Read the model definition and answer for the solid it produces. Units are mm, in the model's axes. A direction names the side the tool comes from. Give positions to 0.01 mm unless a question says otherwise; leave off trailing zeros. Order: outer loops, then holes, each group sorted by start corner. A loop starts at its lowest first (then second) coordinate and runs counter-clockwise, first axis right, second up.
```python
from build123d import *

# Parameters (mm, degrees)
F1_DEPTH      = 300
F3_DEPTH      = 473
F3_DEPTH_BACK = 473
F5_DEPTH      = 473
F5_DEPTH_BACK = 473


with BuildPart() as f1:
    # F0 (on Front) → F1 (new body)
    with BuildSketch(Plane.XZ):
        Polygon((-474, 25), (-474, 0), (473, 0), (473, 25), (472, 25), (472, 1), (-473, 1), (-473, 25), align=None)
    extrude(amount=F1_DEPTH)

    # F2 (on Right) → F3 (join, two sides)
    with BuildSketch(Plane.YZ) as f3_sk:
        with BuildLine():
            Line((-300, -30), (-300, 0))
            Line((-300, 0), (-300, 1))
            ThreePointArc((-300, 1), (-300.707107, 0.707107), (-301, 0))
            Line((-301, 0), (-301, -29))
            Line((-301, -29), (-314, -29))
            Line((-314, -29), (-314, -16))
            Line((-314, -16), (-315, -16))
            Line((-315, -16), (-315, -30))
            Line((-315, -30), (-300, -30))
        make_face()
    extrude(amount=F3_DEPTH)
    extrude(f3_sk.sketch, amount=-F3_DEPTH_BACK)

    # F4 (on Right) → F5 (join, two sides)
    with BuildSketch(Plane.YZ) as f5_sk:
        Polygon((-1, 0), (0, 0), (0, 30), (-10, 30), (-10, 20), (-9, 20), (-9, 29), (-1, 29), align=None)
    extrude(amount=F5_DEPTH)
    extrude(f5_sk.sketch, amount=-F5_DEPTH_BACK)


solid = f1.part
```
1) The part is cut by section B-B on y = -127. Determine the outline of the cut face in (x, z).
Final values:
outline: (-474, 0) - (473, 0) - (473, 25) - (472, 25) - (472, 1) - (-473, 1) - (-473, 25) - (-474, 25) - close
2) The part is cut by section A-A on x = 137. Determine the outline of the cut face in (y, z), and give its area (3 significant figures).
Final values:
outline: (-315, -30) - (-300, -30) - (-300, 0) - (0, 0) - (0, 30) - (-10, 30) - (-10, 20) - (-9, 20) - (-9, 29) - (-1, 29) - (-1, 1) - (-300, 1) arc R1 ccw to (-301, 0) - (-301, -29) - (-314, -29) - (-314, -16) - (-315, -16) - close
area: 405 mm2
3) For a pull along Z with two mould halves and no side action, classify faces 3 (the face through (7, -301, -14)), 4 (the face through (-7, -1, 15)), 5 (the face through (7, -308, -30)) as released by +Z, released by -Z, zero draft, split by the parting line, or undercut.
Final values:
face 3: zero draft
face 4: undercut
face 5: released by -Z
4) Given pin 1 (1.1 mm diameter, centred on x = 4, y = -314.5, fed in from +Z); pin 2 (0.5 mm diameter, centred on x = 472.5, y = -133.5, fed in from +Z); pin 3 (1.1 mm diameter, centred on x = 472.5, z = 7.5, fed in from -Y), each flat-ended and moving along its own axis, determine where each tip first touches the part or whether it passes through.
Final values:
pin 1: stops at z = -16
pin 2: stops at z = 25
pin 3: stops at y = -300
5) A tool of negligible diameter and unlimited length cuts with its end or side. For faces 1 (the face through (-7, 0, 15)), 2 (the face through (7, -300, -15)), from which of +Z, -Z, +X, -X, +Y, -Y can it reach the whole face along a straight path? Write none if from no direction.
Final values:
face 1: +Z, -Z, +X, -X, +Y
face 2: -Z, +X, -X, +Y
6) Consider L1, parallel to X at y = -261.5, z = 24; L2, parallel to Y at x = -75, z = 26; L3, parallel to Y at x = -166, z = -22.5. Determine where each line is inside the solid, lowest interval first.
Final values:
L1: x = -474 to -473, 472 to 473
L2: y = -10 to -9, -1 to 0
L3: y = -315 to -314, -301 to -300
7) The part is cut by section C-C on z = 11. Determine the outline of the cut face in (x, y), and give its area (4 significant figures).
Final values:
outline: (-474, -300) - (-473, -300) - (-473, -1) - (472, -1) - (472, -300) - (473, -300) - (473, 0) - (-474, 0) - close
area: 1,545 mm2
